Verification items for the finished model (mm, model axes). A direction names the side the tool comes from. Coordinates: 2 decimals unless noted, no trailing zeros. Write each loop counter-clockwise with the first axis right and the second up, starting at its lowest first coordinate (ties: lowest second). Pieces come first, ordered by that corner, then holes. Notation, with made-up numbers: (5.25, -28.75) -> (10.25, -28.75) arc R14 cw to (10.25, -2.75) -> close; hole circle Ø1 at (38, 38). An arc over 180 degrees is marked (long way). Answer in a Markdown table with one row per item.
Autodesk Inventor part; units mm, degrees
ref_plane "YZ Plane" through (0, 0, 0) normal (1, 0, 0) x (0, 1, 0)
ref_plane "XZ Plane" through (0, 0, 0) normal (0, 1, 0) x (-1, 0, 0)
ref_plane "XY Plane" through (0, 0, 0) normal (0, 0, 1) x (1, 0, 0)
sketch "Sketch1" plane through (0, 0, 0) normal (0, 1, 0) x (-1, 0, 0)
  line L0 (0, 0) -> (50, 0)
  arc A0 (50, -10) -> (50, 0) centre (50, -5) ccw
  line L1 (50, -10) -> (0, -10)
  line L2 (0, -10) -> (-30, -40)
  line L3 (-30, -40) -> (-60, -10)
  arc A1 (-55.0192, -4.9808) -> (-60, -10) centre (-57.5, -7.5) ccw
  line L4 (-55.0192, -4.9808) -> (-30, -30)
  line L5 (-30, -30) -> (0, 0)
  dimension "d0" = 10
  dimension "d1" = 5
  dimension "d2" = 50
  dimension "d4" = 135
  dimension "d5" = 50
  dimension "d6" = 135
  dimension "d7" = 30
  dimension "d9" = 90
  dimension "d10" = 3.5356
  dimension "d40" = 30
extrude "Extrusion1" add sketch "Sketch1" against normal blind 50
sketch "Sketch2" plane through (-50, 0, 0) normal (0, 0, 1) x (1, 0, 0)
  line L0 (-5, 0) -> (-5, -50)
  line L1 (80, -50) -> (50, -50)
  line L2 (-5, -8) -> (50, -8)
  line L3 (50, -8) -> (50, -50)
  line L4 (50, -50) -> (-5, -50)
  line L5 (-5, -50) -> (-5, -8)
  line L6 (0, 0) -> (50, 0)
  dimension "d13" = 8
extrude "Extrusion2" cut sketch "Sketch2" against normal blind 50
sketch "Sketch3" plane through (-50, -8, 0) normal (0, -1, 0) x (1, 0, 0)
  line L0 (0, 0) -> (50, 0)
  arc A0 (0, 0) -> (0, -10) centre (0, -5) ccw
  circle A1 centre (0, -5) radius 3
  dimension "d19" = 3
extrude "Extrusion3" cut sketch "Sketch3" against normal blind 5
sketch "Sketch4" plane through (-50, -3, -5) normal (0, -1, 0) x (1, 0, 0)
  circle A0 centre (0, 0) radius 0.525
  point P0 (50, 5)
  dimension "d22" = 1.05
extrude "Extrusion4" cut sketch "Sketch4" against normal blind 5
sketch "Sketch5" plane through (30, -50, -40) normal (-0.7071068, 0, -0.7071068) x (-0.7071068, 0, 0.7071068)
  line L0 (42.4264, 42) -> (77.7817, 42)
  line L1 (42.4264, 42) -> (16.7059, 0)
  line L2 (42.4264, 0) -> (0, 0)
  line L3 (16.7059, 0) -> (42.4264, 0)
  line L4 (42.4264, 0) -> (42.4264, 42)
  line L5 (42.4264, 42) -> (42.4264, 0)
  line L6 (7.0711, 50) -> (7.0711, 0)
  line L7 (0, 50) -> (42.4264, 50)
  line L8 (7.0711, 50) -> (42.4264, 50)
  line L9 (42.4264, 50) -> (11.8774, 10.4177)
  line L10 (11.8774, 10.4177) -> (7.0711, 10.4177)
  line L11 (7.0711, 10.4177) -> (7.0711, 50)
  point P0 (49.4975, 50)
  point P1 (7.0711, 10.4177)
  dimension "d41" = 50
extrude "Extrusion5" cut sketch "Sketch5" against normal through all
sketch "Sketch7" plane through (0, -50, 0) normal (0.7071068, 0, 0.7071068) x (0.7071068, 0, -0.7071068)
  line L0 (0, 42) -> (7.0711, 42)
  line L1 (7.0711, 0) -> (7.0711, 42)
  line L2 (0, 42) -> (7.0711, 42)
  line L3 (7.0711, 42) -> (7.0711, 0)
  line L4 (7.0711, 0) -> (0, 0)
  line L5 (0, 0) -> (0, 42)
  point P0 (0, 50)
extrude "Extrusion6" cut sketch "Sketch7" against normal through all
sketch "Sketch8" plane through (55.0192, -50, -4.9808) normal (-0.7071068, 0, 0.7071068) x (0.7071068, 0, 0.7071068)
  line L0 (-42.4536, 10.4177) -> (-42.4536, 50)
  line L1 (-42.4536, 10.4177) -> (3.5084, 10.4177)
  line L2 (3.5084, 10.4177) -> (3.5084, 50.93)
  line L3 (3.5084, 50.93) -> (-42.4536, 50.93)
  line L4 (-42.4536, 50.93) -> (-42.4536, 10.4177)
  point P0 (-35.3825, 50)
  point P1 (-42.4536, 50)
  point P2 (-42.4536, 14.8933)
  point P3 (-42.4536, 14.8933)
extrude "Extrusion7" cut sketch "Sketch8" against normal blind 10
sketch "Sketch9" plane through (30, -50, -30) normal (-0.7071068, 0, 0.7071068) x (0.7071068, 0, 0.7071068)
  line L0 (-7.0711, 0) -> (35.3553, 0)
  line L1 (35.3553, 10.4177) -> (35.3553, 0)
  arc A0 (35.3553, 0) -> (35.3553, 10.4177) centre (33.2861, 5.2088) ccw
  line L2 (38.8909, 10.4177) -> (38.8909, 0)
  line L3 (35.3825, 10.4177) -> (35.3825, 0)
  line L4 (35.3825, 10.4177) -> (38.8909, 10.4177)
  line L5 (35.3553, 0) -> (38.8909, 0)
  line L6 (38.8909, 0) -> (38.8909, 10.4177)
  line L7 (38.8909, 0) -> (35.3553, 0)
  point P0 (0, 50)
  point P1 (35.3825, 10.4068)
  point P2 (38.8909, 5.2088)
  point P3 (35.3825, 0.0109)
extrude "Extrusion8" cut sketch "Sketch9" against normal blind 10 contours L3 L4 L2 A0 | A0 L2 L5 L3
sketch "Sketch10" plane through (30, -50, -30) normal (-0.7071068, 0, 0.7071068) x (0.7071068, 0, 0.7071068)
  line L0 (35.3825, 10.4177) -> (0, 10.4177)
  circle A0 centre (33.2768, 5.2087) radius 2.5
  point P0 (0, 50)
  dimension "d33" = 5.209
  dimension "d34" = 2.5
extrude "Extrusion9" cut sketch "Sketch10" against normal blind 5
sketch "Sketch11" plane through (57.0658, -44.7913, -10.0053) normal (-0.7071068, 0, 0.7071068) x (0.7071068, 0, 0.7071068)
  circle A0 centre (0, 0) radius 1.05
  point P0 (-33.2768, 44.7913)
  dimension "d37" = 1.05
extrude "Extrusion10" cut sketch "Sketch11" against normal blind 11
properties part number "connector"
1. Go/stop test with flat-tipped pins: pin 1 (10 mm diameter, centred on x = -3, z = -11.5, fed in from -Y); pin 2 (4 mm diameter, centred on y = -22.5, z = -8, fed in from +X); pin 3 (6.5 mm diameter, centred on x = -51, z = -4.5, fed in from -Y); pin 4 (3.5 mm diameter, centred on x = -50, z = -5, fed in from -Y). Record where each tip stops, or that it passes through.
Findings below:
| item | result |
|---|---|
| pin 1 | stops at y = -12.57 |
| pin 2 | passes through |
| pin 3 | stops at y = -8 |
| pin 4 | stops at y = -3 |
2. Material ranges on probe 1 along Z at (x, y) = (-50, -6); probe 2 along Y at (x, z) = (-14.5, -4.5); probe 3 along Y at (x, z) = (30, -35.5), recorded low to high. Write a range as from..to.
Findings below:
| item | result |
|---|---|
| probe 1 | z = -10..-8, -2..0 |
| probe 2 | y = -8..0 |
| probe 3 | y = -50..-39.58 |
3. Sectioned sample at B-B, the plane x = -13. Record the cut outline in (y, z).
Findings below:
| item | result |
|---|---|
| outline | (-8, -10) -> (0, -10) -> (0, 0) -> (-8, 0) -> close |
4. Access from +Z, -Z, +X, -X, +Y, -Y to the whole of each face (thin tool, end or side, straight path). Record for faces 4 (the face through (59.81, -46.34, -5.12)), 5 (the face through (-25, -4, -10)), 6 (the face through (16, -27, -16)).
Findings below:
| item | result |
|---|---|
| face 4 | +Z, +X |
| face 5 | -Z, -X, +Y, -Y |
| face 6 | +Z, +Y, -Y |
5. Sectioned sample at C-C, the plane y = -17.5. Record the cut outline in (x, z), and give its area (3 significant figures).
Findings below:
| item | result |
|---|---|
| outline | (4.11, -14.11) -> (9.55, -19.55) -> (14.55, -14.55) -> (9.11, -9.11) -> close |
| area | 54.4 mm² |
6. Release check for a two-part mould opening along Z. For faces 1 (the face through (38, -39.582, -25)), 2 (the face through (-25, -4, 0)), 3 (the face through (-53, -6, -5)) record: released by +Z, released by -Z, zero draft, split by the parting line, or undercut.
Findings below:
| item | result |
|---|---|
| face 1 | zero draft |
| face 2 | released by +Z |
| face 3 | undercut |
7. Sectioned sample at A-A, the plane z = -19. Record the cut outline in (x, y), and give its area (3 significant figures).
Findings below:
| item | result |
|---|---|
| outline | (9, -28.78) -> (19, -40.33) -> (19, -25.65) -> (9, -16.49) -> close; (41, -50) -> (51, -50) -> (51, -39.58) -> (41, -39.58) -> close |
| area | 239 mm² |
